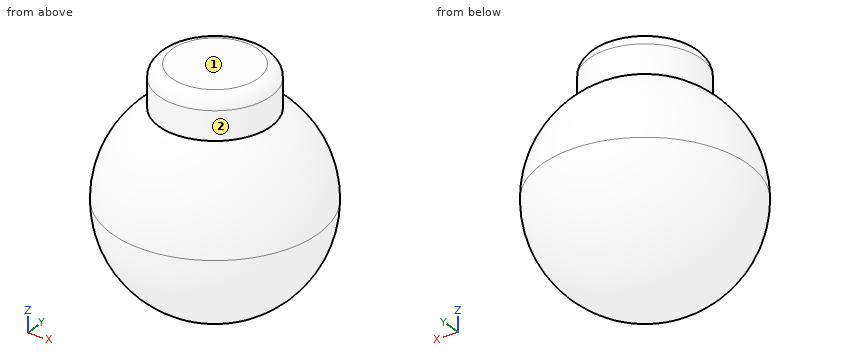
from build123d import *

# Parameters (mm, degrees)
F2_R     = 22.225
F3_DEPTH = 50.8
F4_R     = 5.08


with BuildPart() as f1:
    # F0 (on Front) → F1 (revolve)
    with BuildSketch(Plane.XZ):
        with BuildLine():
            Line((0, -31.9333635271), (0, -40.9301067458))
            ThreePointArc((0, -40.9301067458), (28.9419560347, -28.9419560347), (40.9301067458, 0))
            Line((40.9301067458, 0), (31.9333635271, 0))
            ThreePointArc((31.9333635271, 0), (22.5802978961, -22.5802978961), (0, -31.9333635271))
        make_face()
        with BuildLine():
            Line((31.9333635271, 0), (40.9301067458, 0))
            ThreePointArc((40.9301067458, 0), (28.9419560347, 28.9419560347), (0, 40.9301067458))
            Line((0, 40.9301067458), (0, 31.9333635271))
            ThreePointArc((0, 31.9333635271), (22.5802978961, 22.5802978961), (31.9333635271, 0))
        make_face()
    revolve(axis=Axis((0, 0, 0), (0, 0, -1)))

    # F2 (on Top) → F3 (join)
    with BuildSketch(Plane.XY):
        Circle(F2_R)
    extrude(amount=F3_DEPTH)

    # F4
    f4_edges = [f1.edges().sort_by_distance(p)[0] for p in [
        (-22.225, 0, 50.8),
    ]]
    fillet(f4_edges, radius=F4_R)


solid = f1.part
Read the model definition and answer for the solid it produces. Units are mm, in the model's axes. Face numbers are marked on the shaded views. A direction names the side the tool comes from. Give positions to 0.01 mm unless a question says otherwise; leave off trailing zeros. Write each loop counter-clockwise with the first axis right and the second up, starting at its lowest first coordinate (ties: lowest second). Pieces come first, ordered by that corner, then holes. Notation, with made-up numbers: (-29.75, 52) -> (29.25, 52) arc R22 cw to (29.25, 78) -> close; hole circle Ø1 at (79, -9). An arc over 180 degrees is marked (long way). Answer as a JSON object with one key per item and string values. Group by question number.
1) Consider L1, parallel to X at y = 19, z = 5; L2, parallel to Y at x = -7, z = 13 (3 decimals); L3, parallel to Y at x = 5, z = 6.5. Determine where each line is inside the solid, lowest interval first. Write a range as from..to.
2) Find section D-D (x = 33.5). Write down the section's boundary in (y, z), and give its area (3 significant figures).
3) Find section A-A (x = 0). Write down the section's boundary in (y, z) (3 decimals), and give its area (3 significant figures).
4) Each of these flat-tipped pins is pushed along its axis until it touches: P1, Ø1.5, axis at x = 2.5, y = -3.5, coming from the -Z side; P2, Ø4, axis at y = -9.5, z = 28.5, coming from the +X side; P3, Ø8, axis at x = -5, z = 40.5, coming from the -Y side. Where does it stop, or does it pass through?
5) A tool of negligible diameter and unlimited length cuts with its end or side. For the marked faces 1 and 2, from which of +Z, -Z, +X, -X, +Y, -Y can it reach the whole face along a straight path? Write none if from no direction.
6) Find section C-C (z = 9). Write down the section's boundary in (x, y) (3 decimals).
Values follow:
{
 "1": {"L1": "x = -35.91..-25.17, -11.53..11.53, 25.17..35.91", "L2": "y = -38.174..-28.315, -21.094..21.094, 28.315..38.174", "L3": "y = -40.1..-30.86, -21.66..21.66, 30.86..40.1"},
 "2": {"outline": "circle Ø47.03 at (0, 0)", "area": "1,740 mm2"},
 "3": {"outline": "(-22.225, 34.37) arc R40.93 ccw (long way) to (22.225, 34.37) -> (22.225, 45.72) arc R5.08 ccw to (17.145, 50.8) -> (-17.145, 50.8) arc R5.08 ccw to (-22.225, 45.72) -> close; hole (-22.225, 0) -> (-22.225, 22.93) arc R31.933 ccw (long way) to (22.225, 22.93) -> (22.225, 0) -> close", "area": "3,880 mm2"},
 "4": {"P1": "stops at z = -40.78", "P2": "stops at x = 29.82", "P3": "stops at y = -22.2"},
 "5": {"face 1": "+Z, +X, -X, +Y, -Y", "face 2": "+Z"},
 "6": {"outline": "circle Ø79.857 at (0, 0); circle Ø44.45 at (0, 0); hole circle Ø61.278 at (0, 0)"}
}
